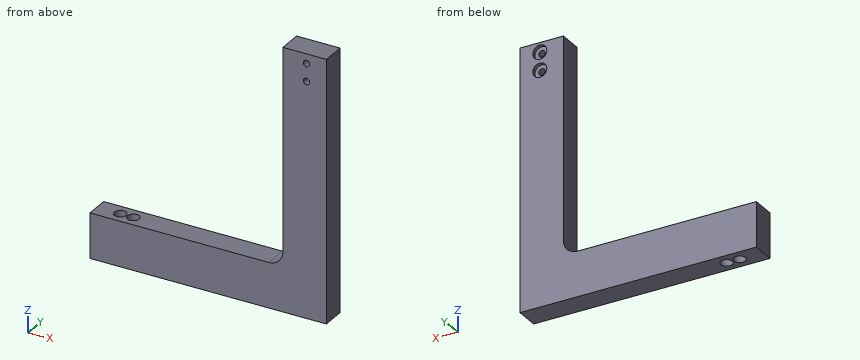
from build123d import *

# Parameters (mm, degrees)
BOSS_EXTRUDE1_DEPTH                                 = 12.7
FILLET1_R                                           = 7.62
CBORE_FOR_5_BINDING_HEAD_MACHINE_SCREW1_D           = 3.4544
CBORE_FOR_5_BINDING_HEAD_MACHINE_SCREW1_DEPTH       = 12.7
CBORE_FOR_5_BINDING_HEAD_MACHINE_SCREW1_CBORE_D     = 7.54126
CBORE_FOR_5_BINDING_HEAD_MACHINE_SCREW1_CBORE_DEPTH = 1.9812
F_1_4_0_25_DIAMETER_HOLE2_D                         = 6.35
F_1_4_0_25_DIAMETER_HOLE2_DEPTH                     = 24.13


with BuildPart() as part:
    # Sketch1 → Boss-Extrude1 (new body)
    with BuildSketch(Plane(origin=(0, 0, 0), x_dir=(1, 0, 0), z_dir=(0, 1, 0))):
        Polygon((-12.7, 39.878), (-116.332, 39.878), (-116.332, 64.008), (10.668, 64.008), (10.668, -76.2), (-12.7, -76.2), align=None)
    extrude(amount=BOSS_EXTRUDE1_DEPTH)

    # Fillet1
    fillet1_edges = [part.edges().sort_by_distance(p)[0] for p in [
        (-12.7, 6.35, -39.878),
    ]]
    fillet(fillet1_edges, radius=FILLET1_R)

    # CBORE for #5 Binding Head Machine Screw1
    with Locations(Plane(origin=(0, 12.7, 0), x_dir=(1, 0, 0), z_dir=(0, 1, 0))):
        with Locations((0, -71.12), (0, -61.560890579)):
            CounterBoreHole(CBORE_FOR_5_BINDING_HEAD_MACHINE_SCREW1_D / 2, CBORE_FOR_5_BINDING_HEAD_MACHINE_SCREW1_CBORE_D / 2, CBORE_FOR_5_BINDING_HEAD_MACHINE_SCREW1_CBORE_DEPTH, depth=CBORE_FOR_5_BINDING_HEAD_MACHINE_SCREW1_DEPTH)

    # 1/4 (0.25) Diameter Hole2
    with Locations(Plane(origin=(0, 0, -64.008), x_dir=(-1, 0, 0), z_dir=(0, 0, -1))):
        with Locations((103.718203887, 6.35), (96.672754807, 6.35)):
            Hole(F_1_4_0_25_DIAMETER_HOLE2_D / 2, depth=F_1_4_0_25_DIAMETER_HOLE2_DEPTH)


solid = part.part
The model under review builds one solid part; all positions refer to its coordinate system, in mm. Round coordinates to 2 decimals unless told otherwise and drop trailing zeros. Write each loop counter-clockwise with the first axis right and the second up, starting at its lowest first coordinate (ties: lowest second). Pieces come first, ordered by that corner, then holes. Notation, with made-up numbers: (26.5, 21.5) -> (36.5, 21.5) arc R22 ccw to (36.5, 33.5) -> close; hole circle Ø8 at (53.25, 21.25). An arc over 180 degrees is marked (long way). Answer as a JSON object with one key per item and string values.
1. We need section D-D on z = 47.5. State the section outline as (x, y) points.
Results found:
{"outline": "(-12.7, 0) -> (10.67, 0) -> (10.67, 12.7) -> (-12.7, 12.7) -> close"}
2. We need section B-B on y = 6.35. State the section outline as (x, z) points.
Results found:
{"outline": "(-116.33, -64.01) -> (-106.89, -64.01) -> (-106.89, -39.88) -> (-116.33, -39.88) -> close; (-100.54, -64.01) -> (-99.85, -64.01) -> (-99.85, -39.88) -> (-100.54, -39.88) -> close; (-93.5, -64.01) -> (10.67, -64.01) -> (10.67, 76.2) -> (-12.7, 76.2) -> (-12.7, -32.26) arc R7.62 cw to (-20.32, -39.88) -> (-93.5, -39.88) -> close; hole circle Ø3.45 at (0, 61.56); hole circle Ø3.45 at (0, 71.12)"}
3. To check wall thickness, follow line 1 along Z through (x, y) = (0, 11.2); line 2 along X through (y, z) = (3.5, -41.5); line 3 along X through (y, z) = (5.5, 71.12). State the ranges of each line that lie inside material, in increasing order.
Results found:
{"line 1": "z = -64.01 to 57.79, 65.33 to 67.35, 74.89 to 76.2", "line 2": "x = -116.33 to -105.12, -102.32 to -98.07, -95.27 to 10.67", "line 3": "x = -12.7 to -1.73, 1.73 to 10.67"}
4. We need section C-C on x = 0. State the section outline as (y, z) points.
Results found:
{"outline": "(0, -64.01) -> (12.7, -64.01) -> (12.7, 57.79) -> (10.72, 57.79) -> (10.72, 59.83) -> (0, 59.83) -> close; (0, 63.29) -> (10.72, 63.29) -> (10.72, 65.33) -> (12.7, 65.33) -> (12.7, 67.35) -> (10.72, 67.35) -> (10.72, 69.39) -> (0, 69.39) -> close; (0, 72.85) -> (10.72, 72.85) -> (10.72, 74.89) -> (12.7, 74.89) -> (12.7, 76.2) -> (0, 76.2) -> close"}
5. We need section A-A on z = 71.12. State the section outline as (x, y) points.
Results found:
{"outline": "(-12.7, 0) -> (-1.73, 0) -> (-1.73, 10.72) -> (-3.77, 10.72) -> (-3.77, 12.7) -> (-12.7, 12.7) -> close; (1.73, 0) -> (10.67, 0) -> (10.67, 12.7) -> (3.77, 12.7) -> (3.77, 10.72) -> (1.73, 10.72) -> close"}
6. Clearance check with flat-ended pins moving along their axes: pin 1 (7 mm diameter, centred on x = 0, z = 71.12, fed in from +Y); pin 2 (2 mm diameter, centred on y = 5, z = 39.5, fed in from -X); pin 3 (6.5 mm diameter, centred on x = -92, y = 5.5, fed in from +Z). State where each tip first meets the part, or that it passes through.
Results found:
{"pin 1": "stops at y = 10.72", "pin 2": "stops at x = -12.7", "pin 3": "stops at z = -39.88"}
